```python
from build123d import *

# Parameters (mm, degrees)
SKETCH_W          = 26.5
SKETCH_H          = 10
SKETCH_W_2        = 24
SKETCH_H_2        = 6.4
PAD_DEPTH         = 20
POCKET_DEPTH      = 5.001
POCKET_DEPTH_BACK = 5.001
SKETCH004_R       = 1.65
PAD001_DEPTH      = 5
SKETCH005_W       = 3.1
SKETCH005_H       = 10
POCKET001_DEPTH   = 3.1
FILLET_R          = 1.2
SKETCH006_W       = 24
SKETCH006_H       = 6.4
POCKET002_DEPTH   = 22
POCKET003_DEPTH   = 3
CHAMFER_SIZE      = 1.79


with BuildPart() as part:
    # Sketch → Pad (new body)
    with BuildSketch(Plane.XY):
        with Locations((18.25, 0)):
            Rectangle(SKETCH_W, SKETCH_H)
        with Locations((17.5, 0)):
            Rectangle(SKETCH_W_2, SKETCH_H_2, mode=Mode.SUBTRACT)
    extrude(amount=PAD_DEPTH)

    # Sketch003 → Pocket (cut, two sides)
    with BuildSketch(Plane.XZ) as pocket_sk:
        with BuildLine():
            Line((5, 0), (5, 10))
            ThreePointArc((15, 20), (7.928932, 17.071068), (5, 10))
            Line((15, 20), (35.5, 20))
            Line((35.5, 20), (35.5, 25))
            Line((35.5, 25), (0, 25))
            Line((0, 25), (0, 0))
            Line((0, 0), (5, 0))
        make_face()
    extrude(amount=-POCKET_DEPTH, mode=Mode.SUBTRACT)
    extrude(pocket_sk.sketch, amount=POCKET_DEPTH_BACK, mode=Mode.SUBTRACT)

    # AdditivePipe: sweep along a path in Sketch002
    with BuildLine(Plane.XZ) as additivepipe_path:
        Line((31.5, 25), (15.000006, 25))
        ThreePointArc((15.000006, 25), (4.393402, 20.606602), (0, 10))
        Line((0, 10), (0, 0))
    # Sketch001 (on Face9 of Pad) → AdditivePipe (sweep)
    with BuildSketch(Plane(origin=(0, 0, 0), x_dir=(1, 0, 0), z_dir=(0, 0, -1))):
        with BuildLine():
            ThreePointArc((5, 5), (0, 10), (-5, 5))
            Line((-5, 5), (-5, -5))
            ThreePointArc((-5, -5), (0, -10), (5, -5))
            Line((5, 5), (5, -5))
        make_face()
        with BuildLine():
            ThreePointArc((3, 5), (0, 8), (-3, 5))
            Line((-3, 5), (-3, -5))
            ThreePointArc((-3, -5), (0, -8), (3, -5))
            Line((3, 5), (3, -5))
        make_face(mode=Mode.SUBTRACT)
    sweep(path=additivepipe_path.line)

    # Sketch004 (on Face2 of AdditivePipe) → Pad001 (join)
    with BuildSketch(Plane(origin=(0, 0, 0), x_dir=(1, 0, 0), z_dir=(0, 0, -1))):
        Polygon((28.522947, 8.5), (26.155811, 12.6), (20.844189, 12.6), (17.495557, 6.8), (9, 6.8), (9, 5), (28.522947, 5), align=None)
        with Locations((23.5, 8)):
            Circle(SKETCH004_R, mode=Mode.SUBTRACT)
    pad001 = extrude(amount=-PAD001_DEPTH)

    # Mirrored: Pad001 across XZ
    add(pad001.mirror(Plane.XZ))

    # Sketch005 (on Face2 of Mirrored) → Pocket001 (cut)
    with BuildSketch(Plane(origin=(0, 0, 0), x_dir=(1, 0, 0), z_dir=(0, 0, -1))):
        with Locations((13.05, 0)):
            Rectangle(SKETCH005_W, SKETCH005_H)
        with Locations((22.55, 0)):
            Rectangle(SKETCH005_W, SKETCH005_H)
    extrude(amount=-POCKET001_DEPTH, mode=Mode.SUBTRACT)

    # Fillet
    fillet_edges = [part.edges().sort_by_distance(p)[0] for p in [
        (11.5, 4.1, 3.1),
        (11.5, -4.1, 3.1),
        (21, -4.1, 3.1),
        (21, 4.1, 3.1),
        (14.6, 4.1, 3.1),
        (14.6, -4.1, 3.1),
        (24.1, -4.1, 3.1),
        (24.1, 4.1, 3.1),
    ]]
    fillet(fillet_edges, radius=FILLET_R)

    # Sketch006 (on Face51 of Fillet) → Pocket002 (cut)
    with BuildSketch(Plane(origin=(0, 0, 0), x_dir=(1, 0, 0), z_dir=(0, 0, -1))):
        with Locations((17.5, 0)):
            Rectangle(SKETCH006_W, SKETCH006_H)
    extrude(amount=-POCKET002_DEPTH, mode=Mode.SUBTRACT)

    # Sketch007 (on Face66 of Pocket002) → Pocket003 (cut)
    with BuildSketch(Plane.XY.offset(5)):
        Polygon((26.733162, -8), (25.116581, -5.2), (21.883419, -5.2), (20.266838, -8), (21.883419, -10.8), (25.116581, -10.8), align=None)
        Polygon((25.116581, 5.2), (26.733162, 8), (25.116581, 10.8), (21.883419, 10.8), (20.266838, 8), (21.883419, 5.2), align=None)
    extrude(amount=-POCKET003_DEPTH, mode=Mode.SUBTRACT)

    # Chamfer
    chamfer_edges = [part.edges().sort_by_distance(p)[0] for p in [
        (9, -6.8, 2.5),
        (9, 6.8, 2.5),
    ]]
    chamfer(chamfer_edges, length=CHAMFER_SIZE)


solid = part.part
```
The model under review builds one solid part; all positions refer to its coordinate system, in mm. A direction names the side the tool comes from. Give positions to 0.01 mm unless a question says otherwise; leave off trailing zeros. Loops run counter-clockwise (first coordinate to the right, second up) from the corner with the lowest first, then second, coordinate; pieces in that order, holes last. Notation, with made-up numbers: (-10.5, -31.5) -> (39.5, -31.5) arc R6 cw to (39.5, -22.5) -> close; hole circle Ø4 at (-29.5, 58.25). An arc over 180 degrees is marked (long way). Use CSV: the item, a comma, the result in double quotes.
1. To check wall thickness, follow probe 1 along Y at (x, z) = (23.5, 1.5); probe 2 along X at (y, z) = (-2.5, 6.5); probe 3 along Z at (x, y) = (26, 7.5). State the ranges of each line that lie inside material, in increasing order. Write a range as from..to.
Result:
probe 1,"y = -12.6..-9.65, -6.35..-5, 5..6.35, 9.65..12.6"
probe 2,"x = -5..-3, 3..5.5, 29.5..31.5"
probe 3,"z = 0..2, 20.67..23.34, 26.66..29.33"
2. For P1, Ø2, axis at y = -7.5, z = 13, coming from the +X side; P2, Ø4, axis at x = 13, z = 1.5, coming from the +Y side; P3, Ø8, axis at y = 1, z = 23, coming from the -X side; P4, Ø12, axis at x = 26.5, z = 10, coming from the -Y side, all flat-tipped, find the tip position at first contact; note any pin that passes through.
Result:
P1,"stops at x = 5.36"
P2,"stops at y = 6.8"
P3,"stops at x = -2.86"
P4,"stops at y = -12.6"
3. The part is to be moulded in two halves that separate along Z. For faces 1 (the face through (11.842, 4.087, 2.739)), 2 (the face through (25, -7, 2)), 3 (the face through (0, -10, 5)), 4 (the face through (2.413, -0.07, 22.867)), say which applies: +Z half, -Z half, draft (parallel to the pull), parting line (faces both ways), or undercut.
Result:
face 1,"-Z half"
face 2,"undercut"
face 3,"draft"
face 4,"undercut"
4. Consider section A-A, the plane y = -2.25. Count the separate pieces of the cut face and the enclosed holes in it, then the cut area to 3 significant figures.
Result:
separate pieces,"3"
enclosed holes,"0"
area,"194 mm²"
5. Consider section C-C, the plane z = 7. Write out the cut boundary in (x, y).
Result:
outline,"(-5, -5) arc R5 ccw to (5, -5) -> (31.5, -5) -> (31.5, 5) -> (5, 5) arc R5 ccw to (-5, 5) -> close; hole (-3, -5) arc R3 ccw to (3, -5) -> (3, 5) arc R3 ccw to (-3, 5) -> close; hole (5.5, -3.2) -> (29.5, -3.2) -> (29.5, 3.2) -> (5.5, 3.2) -> close"
6. Machinability: for faces 5 (the face through (9.91, 5.92, 2.47)), 6 (the face through (9.91, -5.92, 2.47)), 7 (the face through (17, 3.2, 11)), which of the approach directions +Z, -Z, +X, -X, +Y, -Y give a long, thin tool a straight path to every point of the face, cutting with its end or side? Answer none if there is none.
Result:
face 5,"-Z, +Y"
face 6,"-Z, -Y"
face 7,"-Z"
